```python
from build123d import *

# Parameters (mm, degrees)
SKETCH2_W          = 74.9
SKETCH2_H          = 74.9
BASE_DEPTH         = 7.5
SKETCH3_W          = 50.1
SKETCH3_H          = 51.6
SLOT_DEPTH         = 1.6
CUT_EXTRUDE2_DEPTH = 5.9
FILLET1_R          = 30


with BuildPart() as part:
    # Sketch2 → Base (new body)
    with BuildSketch(Plane(origin=(0, 0, 0), x_dir=(1, 0, 0), z_dir=(0, 1, 0))):
        Rectangle(SKETCH2_W, SKETCH2_H)
    extrude(amount=BASE_DEPTH)

    # Sketch3 → Slot (cut)
    with BuildSketch(Plane(origin=(0, 7.5, 0), x_dir=(1, 0, 0), z_dir=(0, 1, 0))):
        Rectangle(SKETCH3_W, SKETCH3_H)
    extrude(amount=-SLOT_DEPTH, mode=Mode.SUBTRACT)

    # Sketch4 → Cut-Extrude2 (cut)
    with BuildSketch(Plane(origin=(0, 5.9, 0), x_dir=(1, 0, 0), z_dir=(0, 1, 0))):
        Polygon((-19.238008182, -25.8), (-19.238008182, 24.800726292), (16.199230682, 24.800726292), (25.05, 15.999956974), (25.05, -14.695394427), (19.490907044, -20.286070377), (19.490907044, -25.8), align=None)
    extrude(amount=-CUT_EXTRUDE2_DEPTH, mode=Mode.SUBTRACT)

    # Fillet1
    fillet1_edges = [part.edges().sort_by_distance(p)[0] for p in [
        (37.45, 3.75, 37.45),
        (-37.45, 3.75, 37.45),
        (-37.45, 3.75, -37.45),
        (37.45, 3.75, -37.45),
    ]]
    fillet(fillet1_edges, radius=FILLET1_R)


solid = part.part
```
Geometry check sheet. Reference: the model listing, model coordinates, mm. A direction names the side the tool comes from. Coordinates: 2 decimals unless noted, no trailing zeros. Order: outer loops, then holes, each group sorted by start corner. A loop starts at its lowest first (then second) coordinate and runs counter-clockwise, first axis right, second up. Notation, with made-up numbers: (27, 39.5) - (36, 39.5) arc R33 ccw to (36, 68.5) - close; hole circle Ø4 at (2, -12.75). An arc over 180 degrees is marked (long way). Answer as a JSON object with one key per item and string values. Group by question number.
Item 1: Sectioned sample at A-A, the plane z = -6. Record the cut outline in (x, y), and give its area (3 significant figures).
Item 2: Sectioned sample at D-D, the plane z = -21. Record the cut outline in (x, y), and give its area (3 significant figures).
Item 3: Tool access check on faces 4 (the face through (22.31, 2.99, 17.45)), 5 (the face through (28.429, 3.802, -28.895)), 6 (the face through (-25.05, 7, 0)). Record the directions out of +Z, -Z, +X, -X, +Y, -Y that give a thin tool (end or side, any length) a straight path to the whole face; none if there is none.
Item 4: Sectioned sample at B-B, the plane x = -12. Record the cut outline in (y, z), and give its area (3 significant figures).
Item 5: Draft check along X on faces 1 (the face through (0, 4, 37.45)), 2 (the face through (28.429, 3.802, 28.895)), 3 (the face through (-19.238, 3, 1)). Enter one of: +X half, -X half, draft (parallel to the pull), parting line (faces both ways), or undercut.
Item 6: Scan lines: probe 1 along X at (y, z) = (3, 5); probe 2 along Z at (x, y) = (-7, 4); probe 3 along X at (y, z) = (2, -20.5). Record each from-to range of solid material in increasing order.
Item 7: Depth check by flat-ended pin: pin 1 Ø3 at (x, z) = (23, 21) entering from +Y; pin 2 Ø4.5 at (y, z) = (4, 23) entering from -X; pin 3 Ø1.5 at (y, z) = (5, 18) entering from +X. Enter the tip coordinate at first touch or a pass-through.
Item 8: Sectioned sample at C-C, the plane y = 5. Record the cut outline in (x, z).
Resolved:
{
 "1": {"outline": "(-37.45, 0) - (-19.24, 0) - (-19.24, 5.9) - (-25.05, 5.9) - (-25.05, 7.5) - (-37.45, 7.5) - close; (25.05, 0) - (37.45, 0) - (37.45, 7.5) - (25.05, 7.5) - close", "area": "220 mm^2"},
 "2": {"outline": "(-34.22, 0) - (-19.24, 0) - (-19.24, 5.9) - (-25.05, 5.9) - (-25.05, 7.5) - (-34.22, 7.5) - close; (20.02, 0) - (34.22, 0) - (34.22, 7.5) - (25.05, 7.5) - (25.05, 5.9) - (20.02, 5.9) - close", "area": "201 mm^2"},
 "3": {"face 4": "+Y, -Y", "face 5": "-Z, +X, +Y, -Y", "face 6": "+Y"},
 "4": {"outline": "(0, -37.1) - (7.5, -37.1) - (7.5, -25.8) - (5.9, -25.8) - (5.9, -24.8) - (0, -24.8) - close; (0, 25.8) - (7.5, 25.8) - (7.5, 37.1) - (0, 37.1) - close", "area": "175 mm^2"},
 "5": {"face 1": "draft", "face 2": "+X half", "face 3": "undercut"},
 "6": {"probe 1": "-37.45 to -19.24, 25.05 to 37.45", "probe 2": "-37.45 to -24.8, 25.8 to 37.45", "probe 3": "-34.46 to -19.24, 20.52 to 34.46"},
 "7": {"pin 1": "y = 5.9", "pin 2": "x = -34.34", "pin 3": "x = 35.8"},
 "8": {"outline": "(-37.45, -7.45) arc R30 ccw to (-7.45, -37.45) - (7.45, -37.45) arc R30 ccw to (37.45, -7.45) - (37.45, 7.45) arc R30 ccw to (7.45, 37.45) - (-7.45, 37.45) arc R30 ccw to (-37.45, 7.45) - close; hole (-19.24, -24.8) - (16.2, -24.8) - (25.05, -16) - (25.05, 14.7) - (19.49, 20.29) - (19.49, 25.8) - (-19.24, 25.8) - close"}
}
